```python
from build123d import *

# Parameters (mm, degrees)
F2_DEPTH    = 12.75
F0_R        = 7
F0_R_2      = 6.5
F0_R_3      = 5.2
F0_R_4      = 5.25
F3_DEPTH    = 25
F4_T1_DEPTH = 37.75
F4_T3_DEPTH = 37.6621075041
F5_R        = 5.207
F6_DEPTH    = 25
F7_SIZE     = 3


# Not quite as in the source:
# - a fillet or chamfer that OpenCascade refuses, or shapes differently, is made with other operations: its cross-section is extruded or revolved along the edge and cut away or added


with BuildPart() as f2:
    # F1 (on Front) → F2 (new body)
    with BuildSketch(Plane.XZ):
        Polygon((270.335, 36.6037324816), (-37.1999023023, 36.6037324816), (-37.1999023023, -4.1193680316), (-65.5964598894, -4.1193680316), (-65.5964598894, -41.3573689769), (-24.4499023023, -41.3573689769), (-24.4499023023, -36.7762675184), (270.335, -36.7762675184), align=None)
    extrude(amount=F2_DEPTH)

    # F0 (on Front) → F3 (cut)
    with BuildSketch(Plane.XZ):
        with BuildLine():
            Line((7.8300976977, 16.6037324816), (-7.7599023023, 16.6037324816))
            ThreePointArc((-7.7599023023, 16.6037324816), (-24.4499023023, -0.0862675184), (-7.7599023023, -16.7762675184))
            Line((-7.7599023023, -16.7762675184), (7.8300976977, -16.7762675184))
            ThreePointArc((7.8300976977, -16.7762675184), (24.5200976977, -0.0862675184), (7.8300976977, 16.6037324816))
        make_face()
        with BuildLine():
            Line((115.045, 16.6037324816), (99.455, 16.6037324816))
            ThreePointArc((99.455, 16.6037324816), (82.765, -0.0862675184), (99.455, -16.7762675184))
            Line((99.455, -16.7762675184), (115.045, -16.7762675184))
            ThreePointArc((115.045, -16.7762675184), (131.735, -0.0862675184), (115.045, 16.6037324816))
        make_face()
        with BuildLine():
            Line((222.295, 16.6037324816), (206.705, 16.6037324816))
            ThreePointArc((206.705, 16.6037324816), (190.015, -0.0862675184), (206.705, -16.7762675184))
            Line((206.705, -16.7762675184), (222.295, -16.7762675184))
            ThreePointArc((222.295, -16.7762675184), (238.985, -0.0862675184), (222.295, 16.6037324816))
        make_face()
        with Locations((36.93, 12.5237324816)):
            Circle(F0_R)
        with Locations((67.822315464, 12.1637324816)):
            Circle(F0_R_2)
        with Locations((67.822315464, -11.5762675184)):
            Circle(F0_R_3)
        with BuildLine():
            Line((-43.9464598894, -16.8693680316), (-47.5964598894, -16.8693680316))
            ThreePointArc((-47.5964598894, -16.8693680316), (-52.8464598894, -22.1193680316), (-47.5964598894, -27.3693680316))
            Line((-47.5964598894, -27.3693680316), (-43.9464598894, -27.3693680316))
            ThreePointArc((-43.9464598894, -27.3693680316), (-38.6964598894, -22.1193680316), (-43.9464598894, -16.8693680316))
        make_face()
        with Locations((144.635, 12.2237324816)):
            Circle(F0_R_2)
        with Locations((144.635, -11.5262675184)):
            Circle(F0_R_4)
        with Locations((176.515, 12.2237324816)):
            Circle(F0_R_2)
        with Locations((176.515, -11.7762675184)):
            Circle(F0_R_2)
        with BuildLine():
            Line((252.38, 16.6037324816), (248.64, 16.6037324816))
            ThreePointArc((248.64, 16.6037324816), (243.435, 11.3987324816), (248.64, 6.1937324816))
            Line((248.64, 6.1937324816), (252.38, 6.1937324816))
            ThreePointArc((252.38, 6.1937324816), (257.585, 11.3987324816), (252.38, 16.6037324816))
        make_face()
        with Locations((252.155, -10.2762675184)):
            Circle(F0_R_2)
    extrude(amount=F3_DEPTH, mode=Mode.SUBTRACT)

    # F4: fillet of radius 5 on 6 edges, made by hand

    # F4_s2 → F4_t1 (cut)
    with BuildSketch(Plane.XZ.offset(-12.5)):
        with BuildLine():
            ThreePointArc((-32.1999023023, 36.6037324816), (-35.7354362082, 35.1392663875), (-37.1999023023, 31.6037324816))
            Line((-37.1999023023, 31.6037324816), (-37.1999023023, 36.6037324816))
            Line((-37.1999023023, 36.6037324816), (-32.1999023023, 36.6037324816))
        make_face()
        with BuildLine():
            ThreePointArc((-60.5964598894, -4.1193680316), (-64.1319937953, -5.5838341257), (-65.5964598894, -9.1193680316))
            Line((-65.5964598894, -9.1193680316), (-65.5964598894, -4.1193680316))
            Line((-65.5964598894, -4.1193680316), (-60.5964598894, -4.1193680316))
        make_face()
        with BuildLine():
            ThreePointArc((-60.5964598894, -41.3573689769), (-64.1319937953, -39.8929028828), (-65.5964598894, -36.3573689769))
            Line((-65.5964598894, -36.3573689769), (-65.5964598894, -41.3573689769))
            Line((-65.5964598894, -41.3573689769), (-60.5964598894, -41.3573689769))
        make_face()
        with BuildLine():
            ThreePointArc((270.335, 31.6037324816), (268.8705339059, 35.1392663875), (265.335, 36.6037324816))
            Line((265.335, 36.6037324816), (270.335, 36.6037324816))
            Line((270.335, 36.6037324816), (270.335, 31.6037324816))
        make_face()
        with BuildLine():
            ThreePointArc((270.335, -31.7762675184), (268.8705339059, -35.3118014243), (265.335, -36.7762675184))
            Line((265.335, -36.7762675184), (270.335, -36.7762675184))
            Line((270.335, -36.7762675184), (270.335, -31.7762675184))
        make_face()
    extrude(amount=F4_T1_DEPTH, mode=Mode.SUBTRACT)

    # F4_s4 → F4_t3 (cut)
    with BuildSketch(Plane.XZ.offset(-12.4560537521)):
        with BuildLine():
            ThreePointArc((-24.4499023023, -36.7762675184), (-26.0481320759, -40.03802739), (-29.4323238031, -41.3573689769))
            Line((-29.4323238031, -41.3573689769), (-24.4499023023, -41.3573689769))
            Line((-24.4499023023, -41.3573689769), (-24.4499023023, -36.7762675184))
        make_face()
    extrude(amount=F4_T3_DEPTH, mode=Mode.SUBTRACT)

    # F5 (on Front) → F6 (cut)
    with BuildSketch(Plane.XZ):
        with Locations((132.714, 24.968)):
            Circle(F5_R)
        with Locations((132.714, -24.968)):
            Circle(F5_R)
        with Locations((81.786, -24.968)):
            Circle(F5_R)
        with Locations((81.786, 24.968)):
            Circle(F5_R)
        with Locations((240.74, -24.968)):
            Circle(F5_R)
        with Locations((-26.24, -24.968)):
            Circle(F5_R)
        with Locations((24.687, 24.968)):
            Circle(F5_R)
        with Locations((189.813, 24.968)):
            Circle(F5_R)
    extrude(amount=F6_DEPTH, mode=Mode.SUBTRACT)

    # F7
    f7_edges = [f2.edges().sort_by_distance(p)[0] for p in [
        (19.48, -12.75, 24.968),
        (-31.447, -12.75, -24.968),
        (76.579, -12.75, 24.968),
        (127.507, -12.75, 24.968),
        (127.507, -12.75, -24.968),
        (76.579, -12.75, -24.968),
        (184.606, -12.75, 24.968),
        (235.533, -12.75, -24.968),
    ]]
    chamfer(f7_edges, length=F7_SIZE)


solid = f2.part
```
Geometry check sheet. Reference: the model listing, model coordinates, mm. A direction names the side the tool comes from. Coordinates: 2 decimals unless noted, no trailing zeros. Write each loop counter-clockwise with the first axis right and the second up, starting at its lowest first coordinate (ties: lowest second). Pieces come first, ordered by that corner, then holes. Notation, with made-up numbers: M 14,25.5 L 18,25.5 A19 ccw 18,43.5 Z; hole C -11.5,39 d3. An arc over 180 degrees is marked long. Answer as a JSON object with one key per item and string values.
1. Go/stop test with flat-tipped pins: pin 1 Ø2 at (y, z) = (-4, 0) entering from -X; pin 2 Ø3 at (x, y) = (251, -6) entering from -Z. Record where each tip stops, or that it passes through.
Answers below:
{"pin 1": "stops at x = -37.2", "pin 2": "stops at z = -36.78"}
2. Section check A-A, the plane x = 36.93. Enter the section's corners in (y, z), plus the area to 3 significant figures.
Answers below:
{"outline": "M -12.75,-36.78 L 0,-36.78 L 0,5.52 L -12.75,5.52 Z; M -12.75,19.52 L 0,19.52 L 0,36.6 L -12.75,36.6 Z", "area": "757 mm²"}
3. Section check C-C, the plane x = 158. Enter the section's corners in (y, z), plus the area to 3 significant figures.
Answers below:
{"outline": "M -12.75,-36.78 L 0,-36.78 L 0,36.6 L -12.75,36.6 Z", "area": "936 mm²"}
4. Section check B-B, the plane y = -5. Give the number of separate pieces and of enclosed holes in the cut face, plus the area to 3 significant figures.
Answers below:
{"separate pieces": "1", "enclosed holes": "21", "area": "17,500 mm²"}
5. Tool access check on faces 3 (the conical face through (137.819, -9.896, 23.36)), 4 (the flat face through (0, -6, -16.776)). Record the directions out of +Z, -Z, +X, -X, +Y, -Y that give a thin tool (end or side, any length) a straight path to the whole face; none if there is none.
Answers below:
{"face 3": "-Y", "face 4": "+Y, -Y"}
6. Scan lines: L1, parallel to Z at x = 133.5, y = -2.5; L2, parallel to X at y = -2.25, z = -4.5 (3 decimals); L3, parallel to Z at x = 77, y = -11.75. Record each from-to range of solid material in increasing order.
Answers below:
{"L1": "z = -36.78 to -30.12, -19.82 to 19.82, 30.12 to 36.6", "L2": "x = -62.51 to -23.856, 23.926 to 83.359, 131.141 to 190.609, 238.391 to 249.174, 255.136 to 270.335", "L3": "z = -36.78 to -30.36, -19.58 to 19.58, 30.36 to 36.6"}
7. Draft check along X on faces 1 (the cylindrical face through (245.707, -4.807, -23.404)), 2 (the flat face through (119, -6, 36.604)). Enter one of: released by +X, released by -X, zero draft, split by the parting line, or undercut.
Answers below:
{"face 1": "undercut", "face 2": "zero draft"}
